The drawing under review shows one solid part. Ordinate dimensions are in mm from its lowest x, y, z. Coordinates: 2 decimals unless noted, no trailing zeros. Write each loop counter-clockwise with the first axis right and the second up, starting at its lowest first coordinate (ties: lowest second). Pieces come first, ordered by that corner, then holes.
Q1. Take a section at A-A (x = 16.4). Give the boundary of the cut face in (y, z), and give its area (3 significant figures).
Q2. Take a section at B-B (z = 80.1). Give the boundary of the cut face in (x, y), and give its area (3 significant figures).
Q3. Insertion check: pin 1 (2.5 mm diameter, centred on x = 126.4, z = 80.1, fed in from +Y). The pin has a flat end and moves straight along its axis. Give the tip position at first contact, or say it passes through.
Q4. For probe 1 along X at (y, z) = (2.45, 80.1); probe 2 along X at (y, z) = (2.25, 21.5), list the stretches that pass through material, from the lowest coordinate up.
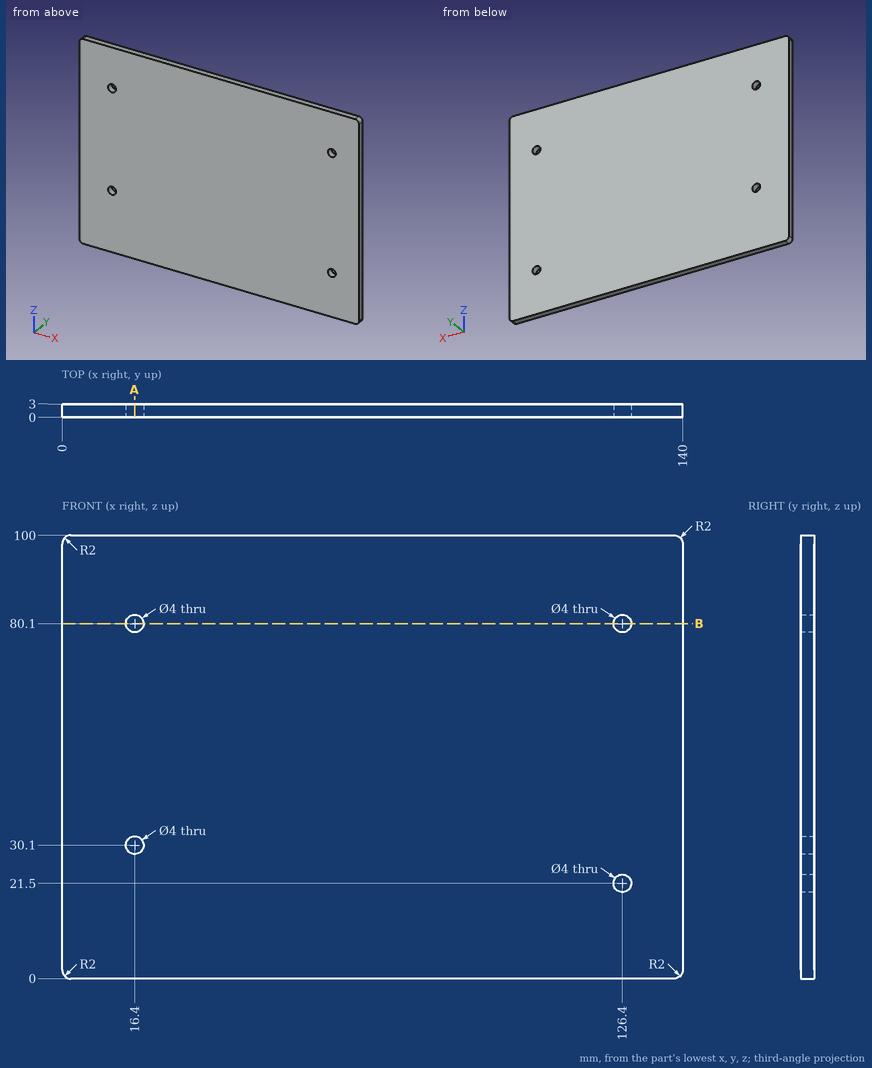
Response:
1. outline: (0, 0) - (3, 0) - (3, 28.1) - (0, 28.1) - close; (0, 32.1) - (3, 32.1) - (3, 78.1) - (0, 78.1) - close; (0, 82.1) - (3, 82.1) - (3, 100) - (0, 100) - close
1. area: 276 mm2
2. outline: (0, 0) - (14.4, 0) - (14.4, 3) - (0, 3) - close; (18.4, 0) - (124.4, 0) - (124.4, 3) - (18.4, 3) - close; (128.4, 0) - (140, 0) - (140, 3) - (128.4, 3) - close
2. area: 396 mm2
3. pin 1: passes through
4. probe 1: x = 0 to 14.4, 18.4 to 124.4, 128.4 to 140
4. probe 2: x = 0 to 124.4, 128.4 to 140
